Geometry: see drawing. Coordinates: mm, zero at the bounding-box minimum. Coordinates: 2 decimals unless noted, no trailing zeros. Order: outer loops, then holes, each group sorted by start corner. A loop starts at its lowest first (then second) coordinate and runs counter-clockwise, first axis right, second up. Notation, with made-up numbers: (59.25, 50.25) -> (97.25, 50.25) arc R15 cw to (97.25, 71.25) -> close; hole circle Ø5 at (-34.75, 9.25). An arc over 180 degrees is marked (long way). Use one line per item in the form item = value.
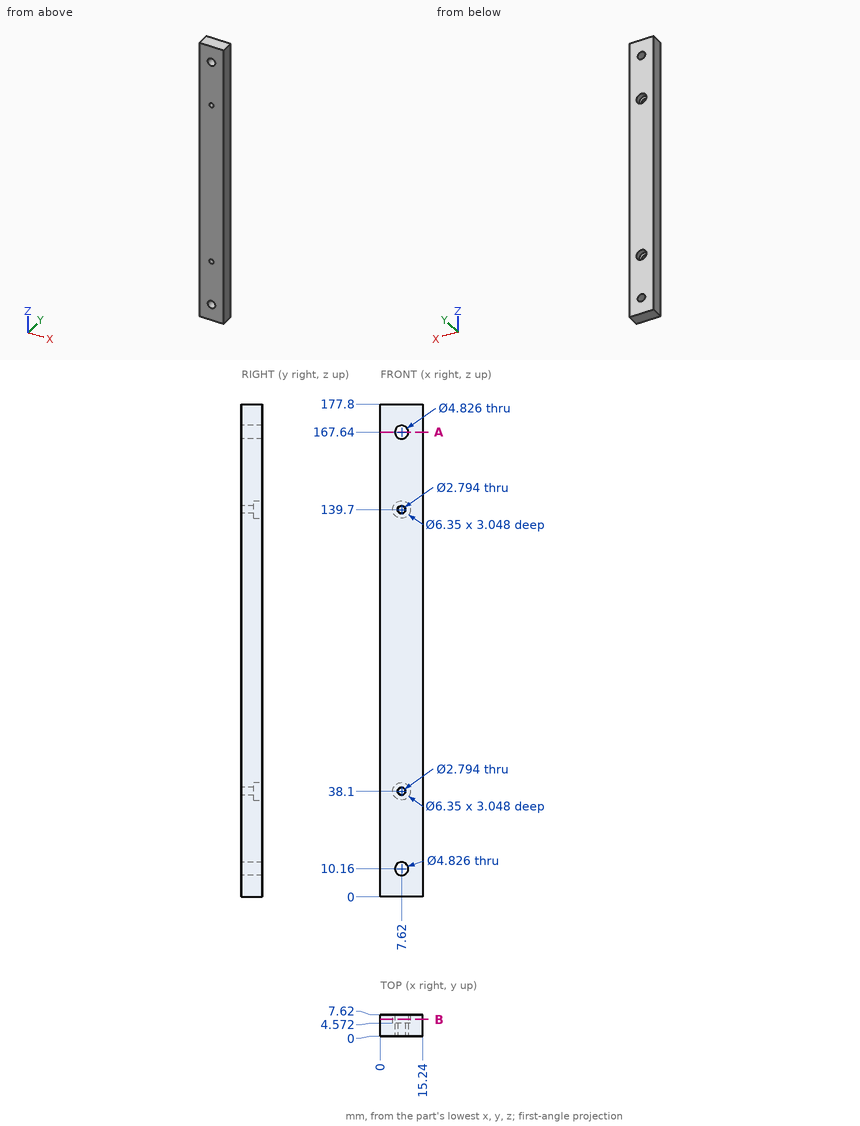
1) Section A-A, the plane z = 167.64. Output: boundary loops of the cut face in (x, y), and give its area (3 significant figures).
Results found:
outline = (0, 0) -> (5.21, 0) -> (5.21, 7.62) -> (0, 7.62) -> close; (10.03, 0) -> (15.24, 0) -> (15.24, 7.62) -> (10.03, 7.62) -> close
area = 79.4 mm2
2) Section B-B, the plane y = 6. Output: boundary loops of the cut face in (x, z) (3 decimals), and give its area (3 significant figures).
Results found:
outline = (0, 0) -> (15.24, 0) -> (15.24, 177.8) -> (0, 177.8) -> close; hole circle Ø6.35 at (7.62, 38.1); hole circle Ø6.35 at (7.62, 139.7); hole circle Ø4.826 at (7.62, 10.16); hole circle Ø4.826 at (7.62, 167.64)
area = 2,610 mm2
3) Contact query for flat-ended pins moving along their axis: P1, Ø3.5, axis at x = 7.62, z = 38.1, coming from the -Y side; P2, Ø4, axis at x = 7.62, z = 10.16, coming from the -Y side; P3, Ø1.9, axis at x = 7.5, z = 141, coming from the +Y side. Output: stop coordinate, or through.
Results found:
P1 = 0
P2 = through
P3 = 4.57
4) Material intervals for probe 1 along Z at (x, y) = (7.62, 5) (3 decimals); probe 2 along Z at (x, y) = (7.62, 2.05); probe 3 along X at (y, z) = (2.75, 167.64), sorted ascending. Write a range as from..to.
Results found:
probe_1 = 0..7.747, 12.573..34.925, 41.275..136.525, 142.875..165.227, 170.053..177.8
probe_2 = 0..7.75, 12.57..36.7, 39.5..138.3, 141.1..165.23, 170.05..177.8
probe_3 = 0..5.21, 10.03..15.24
